Can you work these out from the model? Positions are in its coordinate system, mm. A direction names the side the tool comes from. Coordinates: 2 decimals unless noted, no trailing zeros. Order: outer loops, then holes, each group sorted by start corner. A loop starts at its lowest first (then second) coordinate and runs counter-clockwise, first axis right, second up. Notation, with made-up numbers: (33.25, 73.25) - (47.25, 73.25) arc R32 cw to (47.25, 111.25) - close; hole circle Ø7 at (81.25, 66.5). An arc over 180 degrees is marked (long way). Return JSON: item names as keys, results as strings. Group by question number.
1) Imagine slicing it at D-D (x = -10). Write out the boundary of the cut face in (y, z), and give its area (3 significant figures).
2) Which directions (+Z, -Z, +X, -X, +Y, -Y) give clear straight access to the entire face, cutting with the end or side of a thin tool? Please do faces 4 (the face through (-13, -5, 12)), 5 (the face through (7.215, -2.301, 12.675)), 6 (the face through (19.405, -0.601, 12.675)).
3) If I drill on line 1 along Z through (x, y) = (0, -1.5); line 2 along X through (y, z) = (-4, 18.75) (3 decimals); line 3 along Y through (x, z) = (-0.5, 2.5), over which ranges is the centre line in solid material (lowest first)?
4) For pin 1 Ø2.5 at (x, z) = (-14.5, 15.5) entering from -Y; pin 2 Ø7 at (x, z) = (0, 12.5) entering from +Y; pin 3 Ø6.5 at (x, z) = (2.5, 15.5) entering from -Y; pin 4 Ø1 at (x, z) = (-10.5, 17.5) entering from -Y, each with a flat end and sliding along its axis, tell me the tip position at first contact or that it passes through.
5) If we mould it in two halves opening along X, with no side actions, what happens to faces 1 (the face through (-19.374, -0.57, 12.675)), 2 (the face through (2.01, -1.01, 8.64)), 3 (the face through (-4, 0, 10))? For each: pulls with the +X half, pulls with the -X half, needs draft (parallel to the pull), parting line crosses it, or undercut.
6) Imagine slicing it at C-C (y = -1.5). Write out the boundary of the cut face in (x, z), and give its area (3 significant figures).
7) Imagine slicing it at A-A (x = 0). Write out the boundary of the cut face in (y, z).
```python
from build123d import *

# Parameters (mm, degrees)
F1_DEPTH = 25
F2_R     = 2
F3_R     = 1
F4_R     = 0.8
F5_R     = 4.35
F6_DEPTH = 25


with BuildPart() as f1:
    # F0 (on Top) → F1 (new body)
    with BuildSketch(Plane.XY):
        Polygon((-14.975, -11.3), (-14.975, -8.8), (-17.475, -8.8), (-17.475, -5), (-7.5, -5), (-7.5, -2), (0, -2), (7.5, -2), (7.5, -5), (17.475, -5), (17.475, -8.8), (14.975, -8.8), (14.975, -11.3), (19.975, -11.3), (19.975, 0), (0, 0), (-19.975, 0), (-19.975, -11.3), align=None)
    extrude(amount=F1_DEPTH)

    # F2
    f2_edges = [f1.edges().sort_by_distance(p)[0] for p in [
        (-19.975, 0, 12.5),
        (19.975, 0, 12.5),
        (-19.975, -11.3, 12.5),
        (19.975, -11.3, 12.5),
    ]]
    fillet(f2_edges, radius=F2_R)

    # F3
    f3_edges = [f1.edges().sort_by_distance(p)[0] for p in [
        (7.5, -2, 12.5),
        (-7.5, -2, 12.5),
        (7.5, -5, 12.5),
        (-7.5, -5, 12.5),
        (-14.975, -11.3, 12.5),
        (-14.975, -8.8, 12.5),
        (14.975, -8.8, 12.5),
        (14.975, -11.3, 12.5),
    ]]
    fillet(f3_edges, radius=F3_R)

    # F4
    f4_edges = [f1.edges().sort_by_distance(p)[0] for p in [
        (17.475, -5, 12.5),
        (-17.475, -5, 12.5),
        (-17.475, -8.8, 12.5),
        (17.475, -8.8, 12.5),
    ]]
    fillet(f4_edges, radius=F4_R)

    # F5 (on face) → F6 (cut)
    with BuildSketch(Plane.XZ.offset(2)):
        with Locations((0, 12.5)):
            Circle(F5_R)
    extrude(amount=-F6_DEPTH, mode=Mode.SUBTRACT)


solid = f1.part
```
Calculated:
{
 "1": {"outline": "(-5, 0) - (0, 0) - (0, 25) - (-5, 25) - close", "area": "125 mm2"},
 "2": {"face 4": "+Z, -Z", "face 5": "+Z, -Z, -Y", "face 6": "+Z, -Z, +X, +Y"},
 "3": {"line 1": "0 to 8.15, 16.85 to 25", "line 2": "-19.975 to -7.5, 7.5 to 19.975", "line 3": "-2 to 0"},
 "4": {"pin 1": "y = -11.27", "pin 2": "through", "pin 3": "y = -2", "pin 4": "y = -5"},
 "5": {"face 1": "pulls with the -X half", "face 2": "undercut", "face 3": "needs draft"},
 "6": {"outline": "(-19.91, 0) - (19.91, 0) - (19.91, 25) - (-19.91, 25) - close; hole circle Ø8.7 at (0, 12.5)", "area": "936 mm2"},
 "7": {"outline": "(-2, 0) - (0, 0) - (0, 8.15) - (-2, 8.15) - close; (-2, 16.85) - (0, 16.85) - (0, 25) - (-2, 25) - close"}
}
